```python
from build123d import *

# Parameters (mm, degrees)
SKETCH_3_R          = 4.05
SKETCH_3_R_2        = 4.7
SKETCH_3_W          = 6.2
SKETCH_3_H          = 3
EXTRUDE_1_DEPTH     = 8
SKETCH_4_R          = 6.5
CUT_EXTRUDE_1_DEPTH = 4.5
CUT_EXTRUDE_2_DEPTH = 3
SKETCH_6_R          = 1.6
CUT_EXTRUDE_3_DEPTH = 15
SKETCH_7_R          = 4.05
CUT_EXTRUDE_4_DEPTH = 80.802401326
CHAMFER_1_SIZE      = 2
EXTRUDE_2_DEPTH     = 8


with BuildPart() as part:
    # 草图3 → 凸台-拉伸1 (new body)
    with BuildSketch(Plane.XY):
        with BuildLine():
            Line((43.971143614, 31.160253781), (-7.990379897, 61.160256921))
            ThreePointArc((-7.990379897, 61.160256921), (-15.578570545, 62.159261468), (-21.650634379, 57.500003139))
            Line((-21.650634379, 57.500003139), (-28.355968253, 45.886024187))
            ThreePointArc((-28.355968253, 45.886024187), (-29.495746829, 42.875838443), (-29.620211311, 39.659501706))
            Line((-29.620211311, 39.659501706), (-25.213219189, 4))
            Line((-25.213219189, 4), (-13.416407865, 4))
            ThreePointArc((-13.416407865, 4), (14, 0), (-13.416407865, -4))
            Line((-13.416407865, -4), (-24.224536362, -4))
            Line((-24.224536362, -4), (-22, -22))
            Line((-22, -22), (-22, -30))
            Line((-22, -30), (-7.5, -30))
            Line((-7.5, -30), (-7.5, -22))
            Line((-7.5, -22), (33.97114317, -22))
            Line((33.97114317, -22), (33.97114317, -30))
            Line((33.97114317, -30), (48.97114317, -30))
            Line((48.97114317, -30), (48.97114317, 22.5))
            ThreePointArc((48.97114317, 22.5), (47.631397336, 27.499999778), (43.971143614, 31.160253781))
        make_face()
        with Locations((38.97114317, 22.5)):
            Circle(SKETCH_3_R, mode=Mode.SUBTRACT)
        with Locations((-12.990380341, 52.500003139)):
            Circle(SKETCH_3_R_2, mode=Mode.SUBTRACT)
        with BuildLine():
            Line((-16.3, 17.1), (-14.7, 17.1))
            ThreePointArc((-14.7, 17.1), (-13.1, 15.5), (-14.7, 13.9))
            Line((-14.7, 13.9), (-16.3, 13.9))
            ThreePointArc((-16.3, 13.9), (-17.9, 15.5), (-16.3, 17.1))
        make_face(mode=Mode.SUBTRACT)
        with BuildLine():
            Line((14.7, 17.1), (16.3, 17.1))
            ThreePointArc((16.3, 17.1), (17.9, 15.5), (16.3, 13.9))
            Line((16.3, 13.9), (14.7, 13.9))
            ThreePointArc((14.7, 13.9), (13.1, 15.5), (14.7, 17.1))
        make_face(mode=Mode.SUBTRACT)
        with BuildLine():
            Line((14.7, -13.9), (16.3, -13.9))
            ThreePointArc((16.3, -13.9), (17.9, -15.5), (16.3, -17.1))
            Line((16.3, -17.1), (14.7, -17.1))
            ThreePointArc((14.7, -17.1), (13.1, -15.5), (14.7, -13.9))
        make_face(mode=Mode.SUBTRACT)
        with BuildLine():
            Line((-16.3, -13.9), (-14.7, -13.9))
            ThreePointArc((-14.7, -13.9), (-13.1, -15.5), (-14.7, -17.1))
            Line((-14.7, -17.1), (-16.3, -17.1))
            ThreePointArc((-16.3, -17.1), (-17.9, -15.5), (-16.3, -13.9))
        make_face(mode=Mode.SUBTRACT)
        with Locations((0, -17)):
            Rectangle(SKETCH_3_W, SKETCH_3_H, mode=Mode.SUBTRACT)
        with Locations((28.97114317, -17)):
            Rectangle(SKETCH_3_W, SKETCH_3_H, mode=Mode.SUBTRACT)
    extrude(amount=EXTRUDE_1_DEPTH)

    # 草图4 → 切除-拉伸1 (cut)
    with BuildSketch(Plane(origin=(0, 0, 8), x_dir=(-1, 0, 0), z_dir=(0, 0, -1))):
        with Locations((12.990380341, 52.500003139)):
            Circle(SKETCH_4_R)
    extrude(amount=CUT_EXTRUDE_1_DEPTH, mode=Mode.SUBTRACT)

    # 草图5 → 切除-拉伸2 (cut)
    with BuildSketch(Plane.XY):
        with BuildLine():
            Line((-17.025, 18.55), (-13.975, 18.55))
            ThreePointArc((-13.975, 18.55), (-10.925, 15.5), (-13.975, 12.45))
            Line((-13.975, 12.45), (-17.025, 12.45))
            ThreePointArc((-17.025, 12.45), (-20.075, 15.5), (-17.025, 18.55))
        make_face()
        with BuildLine():
            Line((13.975, 18.55), (17.025, 18.55))
            ThreePointArc((17.025, 18.55), (20.075, 15.5), (17.025, 12.45))
            Line((17.025, 12.45), (13.975, 12.45))
            ThreePointArc((13.975, 12.45), (10.925, 15.5), (13.975, 18.55))
        make_face()
        with BuildLine():
            Line((13.975, -12.45), (17.025, -12.45))
            ThreePointArc((17.025, -12.45), (20.075, -15.5), (17.025, -18.55))
            Line((17.025, -18.55), (13.975, -18.55))
            ThreePointArc((13.975, -18.55), (10.925, -15.5), (13.975, -12.45))
        make_face()
        with BuildLine():
            Line((-17.025, -12.45), (-13.975, -12.45))
            ThreePointArc((-13.975, -12.45), (-10.925, -15.5), (-13.975, -18.55))
            Line((-13.975, -18.55), (-17.025, -18.55))
            ThreePointArc((-17.025, -18.55), (-20.075, -15.5), (-17.025, -12.45))
        make_face()
    extrude(amount=CUT_EXTRUDE_2_DEPTH, mode=Mode.SUBTRACT)

    # 草图6 → 切除-拉伸3 (cut)
    with BuildSketch(Plane.XZ.offset(22)):
        with Locations(Location((0, 4, 0), (0, 0, 270))):
            Circle(SKETCH_6_R)
        with Locations(Location((28.97114317, 4, 0), (0, 0, 270))):
            Circle(SKETCH_6_R)
    extrude(amount=-CUT_EXTRUDE_3_DEPTH, mode=Mode.SUBTRACT)

    # 草图7 → 切除-拉伸4 (cut, through all)
    with BuildSketch(Plane.XY.offset(8)):
        with Locations((38.97114317, 22.5)):
            Circle(SKETCH_7_R)
        with BuildLine():
            Line((-9.216024373, 24.574816528), (-5.72042198, 33.943955438))
            ThreePointArc((-5.72042198, 33.943955438), (-3.469092252, 34.971824328), (-2.441223361, 32.7204946))
            Line((-2.441223361, 32.7204946), (-5.936825754, 23.35135569))
            ThreePointArc((-5.936825754, 23.35135569), (-8.188156046, 22.323485289), (-9.216024373, 24.574816528))
        make_face()
        with BuildLine():
            Line((-18.304089115, 27.965550849), (-14.808486722, 37.334689759))
            ThreePointArc((-14.808486722, 37.334689759), (-12.557156994, 38.362558649), (-11.529288104, 36.111228921))
            Line((-11.529288104, 36.111228921), (-15.024890497, 26.742090011))
            ThreePointArc((-15.024890497, 26.742090011), (-17.276220788, 25.71421961), (-18.304089115, 27.965550849))
        make_face()
    extrude(amount=-CUT_EXTRUDE_4_DEPTH, mode=Mode.SUBTRACT)

    # 倒角1
    chamfer_1_edges = [part.edges().sort_by_distance(p)[0] for p in [
        (48.97114317, -30, 4),
        (33.97114317, -30, 4),
        (-7.5, -30, 4),
        (-22, -30, 4),
    ]]
    chamfer(chamfer_1_edges, length=CHAMFER_1_SIZE)

    # 草图9 → 凸台-拉伸2 (add)
    with BuildSketch(Plane.XY.offset(8)):
        Polygon((2.85, -15.9), (-2.85, -15.9), (-2.85, -18.5), (-3.1, -18.5), (-3.1, -15.5), (3.1, -15.5), (3.1, -18.5), (2.85, -18.5), align=None)
        Polygon((31.82114317, -15.9), (26.12114317, -15.9), (26.12114317, -18.5), (25.87114317, -18.5), (25.87114317, -15.5), (32.07114317, -15.5), (32.07114317, -18.5), (31.82114317, -18.5), align=None)
    extrude(amount=-EXTRUDE_2_DEPTH)


solid = part.part
```
Source: CAD feature listing. Evaluate the final solid. Frame: model axes, mm. A direction names the side the tool comes from. Give positions to 0.01 mm unless a question says otherwise; leave off trailing zeros. Write each loop counter-clockwise with the first axis right and the second up, starting at its lowest first coordinate (ties: lowest second). Pieces come first, ordered by that corner, then holes.
1. Material intervals for line 1 along Z through (x, y) = (0, -14.2); line 2 along X through (y, z) = (-19.7, 4); line 3 along Y through (x, z) = (16, 1), sorted ascending.
2. Access query for faces 4 (the face through (-0.97, -20.27, 5.27)), 5 (the face through (-2.85, -17, 4)), 6 (the face through (13, -22, 4)). Directions: +Z, -Z, +X, -X, +Y, -Y. A direction counts if a zero-diameter tool reaches every point of the face in a straight line with its end or side. Return the directions, or none.
3. Pull-direction query (X, two-part tool) for faces 1 (the face through (41, -30, 4)), 2 (the face through (47.668, 27.436, 3.944)), 3 (the face through (-15.4, 13.5, 3)); classes: +X half, -X half, draft (parallel to the pull), parting line (faces both ways), or undercut.
4. Section query D-D (y = 15.5). Return the cut outline in (x, z) (3 decimals), then the cut area to 3 significant figures.
5. Section query A-A (y = -9). Return the cut outline in (x, z), then the cut area to 3 significant figures.
6. Section query C-C (x = 0). Return the cut outline in (y, z).
7. First-contact query: pin 1 (1.3 mm diameter, centred on x = 15.5, z = 6, fed in from +Y); pin 2 (4.5 mm diameter, centred on x = 1, z = 3, fed in from -Y); pin 3 (4 mm diameter, centred on x = -19.5, z = 2.5, fed in from +Y). Flat tips, straight axial feed; report the tip coordinate or a pass-through.
8. Section query B-B (y = 30). Return the cut outline in (x, z), then the cut area to 3 significant figures.
Output values:
1. line 1: z = 0 to 2.4, 5.6 to 8
1. line 2: x = -22.28 to -1.6, 1.6 to 27.37, 30.57 to 48.97
1. line 3: y = -22 to -18.55, -12.45 to 12.45, 18.55 to 47.31
2. face 4: -Y
2. face 5: +Z, -Z
2. face 6: +Z, -Z, -Y
3. face 1: draft
3. face 2: +X half
3. face 3: undercut
4. outline: (-26.634, 0) - (-20.075, 0) - (-20.075, 3) - (-17.9, 3) - (-17.9, 8) - (-26.634, 8) - close; (-13.1, 3) - (-10.925, 3) - (-10.925, 0) - (10.925, 0) - (10.925, 3) - (13.1, 3) - (13.1, 8) - (-13.1, 8) - close; (17.9, 3) - (20.075, 3) - (20.075, 0) - (48.971, 0) - (48.971, 8) - (17.9, 8) - close
4. area: 502 mm2
5. outline: (-23.61, 0) - (-10.72, 0) - (-10.72, 8) - (-23.61, 8) - close; (10.72, 0) - (48.97, 0) - (48.97, 8) - (10.72, 8) - close; hole circle Ø3.2 at (28.97, 4)
5. area: 401 mm2
6. outline: (-22, 0) - (-18.5, 0) - (-18.5, 2.4) - (-22, 2.4) - close; (-22, 5.6) - (-18.5, 5.6) - (-18.5, 8) - (-22, 8) - close; (-15.9, 0) - (-14, 0) - (-14, 2.4) - (-15.5, 2.4) - (-15.5, 5.6) - (-14, 5.6) - (-14, 8) - (-15.9, 8) - close; (14, 0) - (56.55, 0) - (56.55, 8) - (14, 8) - close
7. pin 1: stops at y = 47.97
7. pin 2: stops at y = -22
7. pin 3: stops at y = 61.43
8. outline: (-28.43, 0) - (-17.55, 0) - (-17.55, 8) - (-28.43, 8) - close; (-13.81, 0) - (-7.19, 0) - (-7.19, 8) - (-13.81, 8) - close; (-3.46, 0) - (45.59, 0) - (45.59, 8) - (-3.46, 8) - close
8. area: 532 mm2
